Check sheet for the modelled part. Datum: model origin and axes. Units: mm. Face numbers are marked on the shaded views. Give positions to 0.01 mm unless a question says otherwise; leave off trailing zeros. Write each loop counter-clockwise with the first axis right and the second up, starting at its lowest first coordinate (ties: lowest second). Pieces come first, ordered by that corner, then holes. Notation, with made-up numbers: M -35,10.25 L -4,10.25 A8 cw -4,24.25 Z; hole C 34,-13 d2. An arc over 180 degrees is marked long. Write each question's results on one line, items separated by ' | '. Start each with the question number.
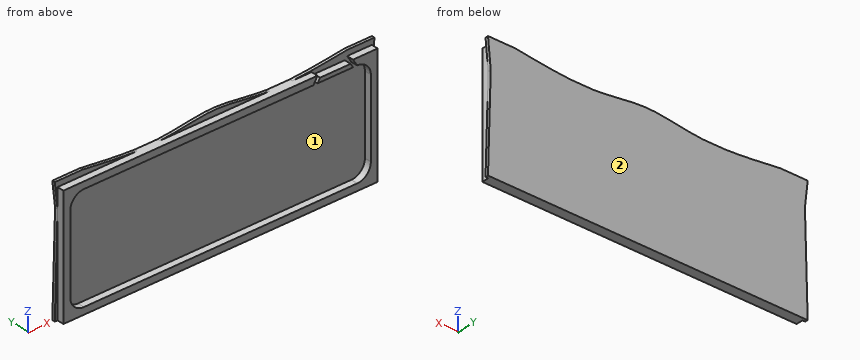
from build123d import *

# Parameters (mm, degrees)
F0_W     = 584.2
F0_H     = 219.71
F1_DEPTH = 5.334
F2_W     = 558.8
F2_H     = 194.31
F3_DEPTH = 12.7
F4_R     = 25.4
F6_DEPTH = 12.7
F8_DEPTH = 5.334


# Not quite as in the source:
# - a feature names something its author has since deleted; it is built from what else it names


with BuildPart() as f1:
    # F0 (on Front) → F1 (new body)
    with BuildSketch(Plane.XZ):
        with Locations((-292.1, 109.855)):
            Rectangle(F0_W, F0_H)
    extrude(amount=F1_DEPTH)

    # F2 (on face) → F3 (join)
    with BuildSketch(Plane.XZ.offset(5.334)):
        Polygon((0, 219.71), (-6.35, 219.71), (-577.85, 219.71), (-584.2, 219.71), (-584.2, 0), (0, 0), align=None)
        with Locations((-292.1, 109.855)):
            Rectangle(F2_W, F2_H, mode=Mode.SUBTRACT)
    extrude(amount=F3_DEPTH)

    # F4
    f4_edges = [f1.edges().sort_by_distance(p)[0] for p in [
        (-571.5, -11.684, 207.01),
        (-12.7, -11.684, 207.01),
        (-12.7, -11.684, 12.7),
        (-571.5, -11.684, 12.7),
    ]]
    fillet(f4_edges, radius=F4_R)

    # F5 (on face) → F6 (cut)
    with BuildSketch(Plane.XZ.offset(18.034)):
        Polygon((-104.14, 219.71), (-111.76, 219.71), (-119.38, 207.01), (-111.76, 207.01), (-107.2320166854, 214.5566388576), align=None)
        Polygon((-38.1, 207.01), (-45.72, 219.71), (-53.34, 219.71), (-50.2479833146, 214.5566388576), (-45.72, 207.01), align=None)
        Polygon((-53.34, 219.71), (-104.14, 219.71), (-107.2320166854, 214.5566388576), (-50.2479833146, 214.5566388576), align=None)
    extrude(amount=-F6_DEPTH, mode=Mode.SUBTRACT)

    # F7 (on face) → F8 (join)
    with BuildSketch(Plane(origin=(0, 0, 0), x_dir=(-1, 0, 0), z_dir=(0, 1, 0))):
        with BuildLine():
            Line((-5.08, 229.87), (0, 176.1275827885))
            Line((0, 176.1275827885), (0, 219.71))
            Line((0, 219.71), (148.0852009026, 219.71))
            add(Edge.make_bspline(
                [(148.0852009026, 219.71), (115.3779899576, 221.1840971885), (80.5489949788, 225.5270485943), (45.72, 229.87)],
                knots=[0.812101374, 0.812101374, 0.812101374, 0.812101374, 1, 1, 1, 1], degree=3))
            Line((45.72, 229.87), (-5.08, 229.87))
        make_face()
        with BuildLine():
            add(Edge.make_bspline(
                [(393.7, 219.71), (356.8171998762, 221.731425099), (324.4585999381, 229.87), (292.1, 229.87)],
                knots=[0.2719218593, 0.2719218593, 0.2719218593, 0.2719218593, 0.5, 0.5, 0.5, 0.5], degree=3))
            add(Edge.make_bspline(
                [(292.1, 229.87), (259.7414000619, 229.87), (227.3828001238, 221.731425099), (190.5, 219.71)],
                knots=[0.5, 0.5, 0.5, 0.5, 0.7280781407, 0.7280781407, 0.7280781407, 0.7280781407], degree=3))
            Line((190.5, 219.71), (393.7, 219.71))
        make_face()
        Polygon((584.2, 183.2547038794), (584.2, 0), (589.28, 0), align=None)
        with BuildLine():
            Line((584.2, 219.71), (584.2, 183.2547038794))
            Line((584.2, 183.2547038794), (589.28, 229.87))
            Line((589.28, 229.87), (538.48, 229.87))
            add(Edge.make_bspline(
                [(538.48, 229.87), (503.6510050212, 225.5270485943), (468.8220100424, 221.1840971885), (436.1147990974, 219.71)],
                knots=[0, 0, 0, 0, 0.187898626, 0.187898626, 0.187898626, 0.187898626], degree=3))
            Line((436.1147990974, 219.71), (584.2, 219.71))
        make_face()
        Polygon((-5.08, 0), (0, 0), (0, 176.1275827885), align=None)
    extrude(amount=-F8_DEPTH)


solid = f1.part
Q1. Section check B-B on z = 19.5. Record the boundary of the cut face in (x, y), plus the area to 3 significant figures.
Q2. Scan lines: L1, parallel to Z at x = -398.5, y = -8.5; L2, parallel to X at y = -13.5, z = 158; L3, parallel to Y at x = -174, z = 164. Record each from-to range of solid material in increasing order.
Q3. Section check C-C on z = 54. Record the boundary of the cut face in (x, y).
Q4. Release check for a two-part mould opening along X. For the marked faces 1 and 2 record: pulls with the +X half, pulls with the -X half, needs draft (parallel to the pull), parting line crosses it, or undercut.
Q5. Section check A-A on y = -9. Record the boundary of the cut face in (x, z), plus the area to 3 significant figures.
Q6. Depth check by flat-ended pin: pin 1 Ø8 at (y, z) = (-11, 43.5) entering from +X; pin 2 Ø5 at (x, z) = (-267, 224.5) entering from -Y; pin 3 Ø5.5 at (x, y) = (-421.5, -9) entering from +Z. Enter the tip coordinate at first touch or a pass-through.
Check result:
1) outline: M -588.74,-5.33 L -584.2,-5.33 L -584.2,-18.03 L -563.4,-18.03 L -563.4,-5.33 L -20.8,-5.33 L -20.8,-18.03 L 0,-18.03 L 0,-5.33 L 4.52,-5.33 L 4.52,0 L -588.74,0 Z | area: 3,690 mm^2
2) L1: 0 to 12.7, 207.01 to 219.71 | L2: -584.2 to -571.5, -12.7 to 0 | L3: -5.33 to 0
3) outline: M -587.78,-5.33 L -584.2,-5.33 L -584.2,-18.03 L -571.5,-18.03 L -571.5,-5.33 L -12.7,-5.33 L -12.7,-18.03 L 0,-18.03 L 0,-5.33 L 3.52,-5.33 L 3.52,0 L -587.78,0 Z
4) face 1: undercut | face 2: needs draft
5) outline: M -584.2,0 L 0,0 L 0,219.71 L -45.72,219.71 L -38.1,207.01 A25.4 cw -12.7,181.61 L -12.7,38.1 A25.4 cw -38.1,12.7 L -546.1,12.7 A25.4 cw -571.5,38.1 L -571.5,181.61 A25.4 cw -546.1,207.01 L -119.38,207.01 L -111.76,219.71 L -584.2,219.71 Z; M -111.76,207.01 L -45.72,207.01 L -50.25,214.56 L -107.23,214.56 Z | area: 19,900 mm^2
6) pin 1: x = 0 | pin 2: y = -5.33 | pin 3: z = 219.71
